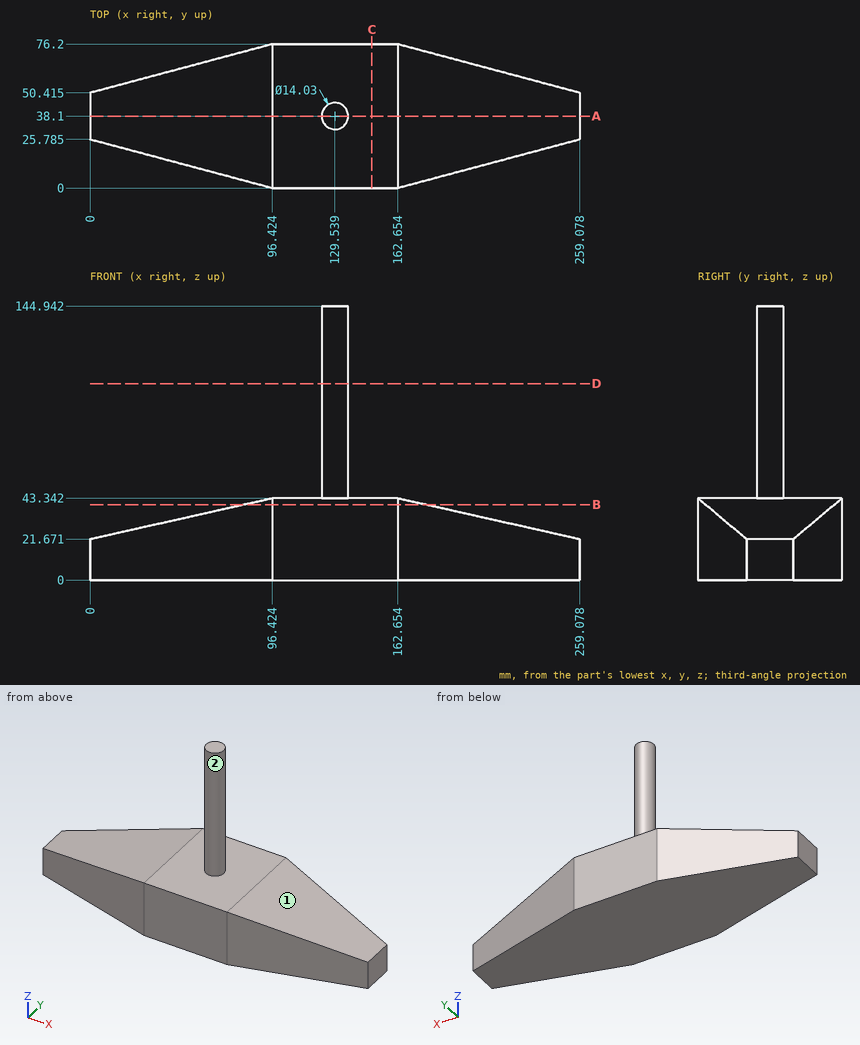
For this review, use the dimensioned drawing (mm, ordinates from the lowest corner) and the shaded views. A direction names the side the tool comes from. Round coordinates to 2 decimals unless told otherwise and drop trailing zeros. Order: outer loops, then holes, each group sorted by start corner. A loop starts at its lowest first (then second) coordinate and runs counter-clockwise, first axis right, second up. Notation, with made-up numbers: (60, -36) -> (119, -36) arc R35 ccw to (119, -2) -> close; hole circle Ø8 at (38.25, -37.5). An arc over 180 degrees is marked (long way). One line per item, written item: value. Start each with the question number.
Q1. Wall thickness on line 1 (Z direction, x = 107, y = 16); line 2 (Z direction, x = 79.5, y = 42); line 3 (Y direction, x = 43.5, z = 16.5): over which ranges is each line inside the solid? List them lowest first.
Q2. Machinability: for the marked faces 1 and 2, which of the approach directions +Z, -Z, +X, -X, +Y, -Y give a long, thin tool a straight path to every point of the face, cutting with its end or side? Answer none if there is none.
Q3. Take a section at C-C (x = 149). Write out the cut boundary in (y, z), and give its area (3 significant figures).
Q4. Take a section at A-A (y = 38.1). Write out the cut boundary in (x, z), and give its area (3 significant figures).
Q5. Take a section at B-B (z = 40). Write out the cut boundary in (x, y).
Q6. Take a section at D-D (z = 104). Write out the cut boundary in (x, y) (1 decimal), and give its area (3 significant figures).
Q7. Clearance check with flat-ended pins moving along their axes: pin 1 Ø1.5 at (x, y) = (85, 14) entering from +Z; pin 2 Ø10 at (x, y) = (229.5, 13) entering from +Z (1 decimal); pin 3 Ø6 at (y, z) = (34, 83) entering from +X. State where each tip first meets the part, or that it passes through.
Reported:
1. line 1: z = 0 to 43.34
1. line 2: z = 0 to 39.54
1. line 3: y = 14.15 to 62.05
2. face 1: +Z, +X, +Y, -Y
2. face 2: +Z
3. outline: (0, 0) -> (76.2, 0) -> (76.2, 43.34) -> (0, 43.34) -> close
3. area: 3,300 mm2
4. outline: (0, 0) -> (259.08, 0) -> (259.08, 21.67) -> (162.65, 43.34) -> (136.55, 43.34) -> (136.55, 144.94) -> (122.52, 144.94) -> (122.52, 43.34) -> (96.42, 43.34) -> (0, 21.67) -> close
4. area: 10,600 mm2
5. outline: (81.55, 3.98) -> (96.42, 0) -> (162.65, 0) -> (177.52, 3.98) -> (177.52, 72.22) -> (162.65, 76.2) -> (96.42, 76.2) -> (81.55, 72.22) -> close
6. outline: circle Ø14 at (129.5, 38.1)
6. area: 155 mm2
7. pin 1: stops at z = 40.94
7. pin 2: stops at z = 29
7. pin 3: stops at x = 136.47
